Geometry check sheet. Reference: the model listing, model coordinates, mm. A direction names the side the tool comes from. Coordinates: 2 decimals unless noted, no trailing zeros. Write each loop counter-clockwise with the first axis right and the second up, starting at its lowest first coordinate (ties: lowest second). Pieces come first, ordered by that corner, then holes. Notation, with made-up numbers: (5.25, 9) -> (43.25, 9) arc R25 ccw to (43.25, 23) -> close; hole circle Ø1 at (-24.5, 34.25). An arc over 180 degrees is marked (long way). Answer in a Markdown table with one row per item. Add a question column.
1. Cross-section at A-A on z = 0. Give the number of separate pieces and of enclosed holes in the cut face, and give its area (3 significant figures).
2. Cross-section at D-D on y = -6.75. Record the cut outline in (x, z), and give its area (3 significant figures).
3. Cross-section at C-C on y = -1. Record the cut outline in (x, z), and give its area (3 significant figures).
4. Depth check by flat-ended pin: P1, Ø2, axis at y = -11, z = -4, coming from the -X side; P2, Ø1, axis at y = -1.5, z = 4, coming from the +X side; P3, Ø8, axis at x = 11, z = -3, coming from the -Y side. Enter the tip coordinate at first touch or a pass-through.
5. Mould release check, pull along Z, two halves, no side actions. Record for faces 3 (the cylindrical face through (-23.75, -1.97, 0.09)), 4 (the flat face through (-1.42, -13, -3.92)), 5 (the cylindrical face through (-0.867, -6.409, -3.905)): pulls with the +Z half, pulls with the -Z half, needs draft (parallel to the pull), parting line crosses it, or undercut.
6. Cross-section at B-B on x = 0. Record the cut outline in (y, z).
7. Scan lines: L1, parallel to X at y = -2.5, z = -1.5; L2, parallel to Z at x = 0, y = -7; L3, parallel to Y at x = 12, z = -8. Record each from-to range of solid material in increasing order. Write a range as from..to.
8. Set-up check for faces 1 (the flat face through (13.186, -1.972, -8.589)), 2 (the cylindrical face through (6.466, -10.986, -2.681)): record each of +Z, -Z, +X, -X, +Y, -Y from which the full face is reachable in a straight line by a thin tool's end or side.
```python
from build123d import *

# Parameters (mm, degrees)
F0_R     = 2.5
F0_R_2   = 4
F1_DEPTH = 4
F2_R     = 11
F2_R_2   = 4
F3_DEPTH = 5
F4_R     = 7
F4_R_2   = 4
F5_DEPTH = 4
F6_R     = 1


with BuildPart() as f1:
    # F0 (on Front) → F1 (new body)
    with BuildSketch(Plane.XZ):
        with BuildLine():
            Line((-20.660959, -4.943407), (-5.917808, -12.133818))
            ThreePointArc((-5.917808, -12.133818), (0, -13.5), (5.917808, -12.133818))
            Line((5.917808, -12.133818), (20.660959, -4.943407))
            ThreePointArc((20.660959, -4.943407), (23.75, 0), (20.660959, 4.943407))
            Line((20.660959, 4.943407), (5.917808, 12.133818))
            ThreePointArc((5.917808, 12.133818), (0, 13.5), (-5.917808, 12.133818))
            Line((-5.917808, 12.133818), (-20.660959, 4.943407))
            ThreePointArc((-20.660959, 4.943407), (-23.75, 0), (-20.660959, -4.943407))
        make_face()
        with Locations((-18.25, 0)):
            Circle(F0_R, mode=Mode.SUBTRACT)
        Circle(F0_R_2, mode=Mode.SUBTRACT)
        with Locations((18.25, 0)):
            Circle(F0_R, mode=Mode.SUBTRACT)
    extrude(amount=F1_DEPTH)

    # F2 (on face) → F3 (join)
    with BuildSketch(Plane.XZ.offset(4)):
        Circle(F2_R)
        Circle(F2_R_2, mode=Mode.SUBTRACT)
    extrude(amount=F3_DEPTH)

    # F4 (on face) → F5 (join)
    with BuildSketch(Plane.XZ.offset(9)):
        Circle(F4_R)
        Circle(F4_R_2, mode=Mode.SUBTRACT)
    extrude(amount=F5_DEPTH)

    # F6
    f6_edges = [f1.edges().sort_by_distance(p)[0] for p in [
        (-11, -9, 0),
        (-7, -9, 0),
        (-11, -4, 0),
        (-7, -13, 0),
    ]]
    fillet(f6_edges, radius=F6_R)


solid = f1.part
```
Results found:
| question | item | result |
|---|---|---|
| 1 | separate pieces | 4 |
| 1 | enclosed holes | 0 |
| 1 | area | 212 mm^2 |
| 2 | outline | circle Ø22 at (0, 0); hole circle Ø8 at (0, 0) |
| 2 | area | 330 mm^2 |
| 3 | outline | (-20.66, -4.94) -> (-5.92, -12.13) arc R13.5 ccw to (5.92, -12.13) -> (20.66, -4.94) arc R5.5 ccw to (20.66, 4.94) -> (5.92, 12.13) arc R13.5 ccw to (-5.92, 12.13) -> (-20.66, 4.94) arc R5.5 ccw to start; hole circle Ø5 at (-18.25, 0); hole circle Ø8 at (0, 0); hole circle Ø5 at (18.25, 0) |
| 3 | area | 767 mm^2 |
| 4 | P1 | stops at x = -6.32 |
| 4 | P2 | stops at x = 22.49 |
| 4 | P3 | stops at y = -9.2 |
| 5 | face 3 | parting line crosses it |
| 5 | face 4 | needs draft |
| 5 | face 5 | undercut |
| 6 | outline | (-13, -6) arc R1 ccw to (-12, -7) -> (-10, -7) arc R1 cw to (-9, -8) -> (-9, -10) arc R1 ccw to (-8, -11) -> (-5, -11) arc R1 cw to (-4, -12) -> (-4, -13.5) -> (0, -13.5) -> (0, -4) -> (-13, -4) -> close; (-13, 4) -> (0, 4) -> (0, 13.5) -> (-4, 13.5) -> (-4, 12) arc R1 cw to (-5, 11) -> (-8, 11) arc R1 ccw to (-9, 10) -> (-9, 8) arc R1 cw to (-10, 7) -> (-12, 7) arc R1 ccw to (-13, 6) -> close |
| 7 | L1 | x = -23.54..-20.25, -16.25..-3.71, 3.71..16.25, 20.25..23.54 |
| 7 | L2 | z = -11..-4, 4..11 |
| 7 | L3 | y = -4..0 |
| 8 | face 1 | -Z, +X, +Y, -Y |
| 8 | face 2 | -Y |
